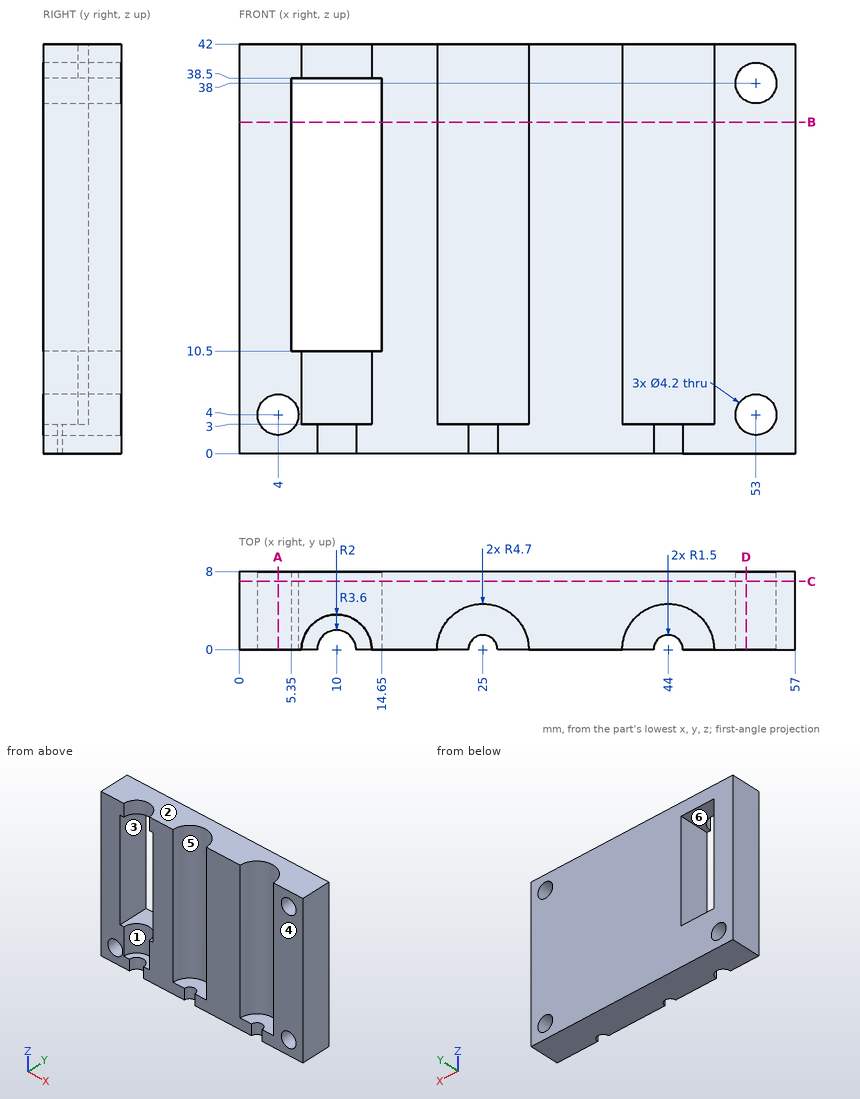
Print and shaded views of the part. All mm, measured from the part's lowest x, y and z. A direction names the side the tool comes from. Round coordinates to 2 decimals unless told otherwise and drop trailing zeros. Write each loop counter-clockwise with the first axis right and the second up, starting at its lowest first coordinate (ties: lowest second). Pieces come first, ordered by that corner, then holes.
(1) Probe line 1 along X through (y, z) = (5.5, 38); line 2 along X through (y, z) = (5, 4); line 3 along X through (y, z) = (2.25, 4). List the from-to ranges inside material, lowest first.
(2) Mould opens along Z. For the marked faces 1, 2 and 3 say: pulls with the +Z half, pulls with the -Z half, needs draft (parallel to the pull), parting line crosses it, or undercut.
(3) Slice it at D-D, the plane x = 52. Write the cut outline in (y, z).
(4) 3-axis set-ups, long thin cutter, end or side, ignore diameter. For the marked faces 4, 5 and 6: which of +Z, -Z, +X, -X, +Y, -Y reach the whole face in a straight line?
(5) Slice it at B-B, the plane z = 34. Write the cut outline in (x, y).
(6) Slice it at A-A, the plane x = 4. Write the cut outline in (y, z).
(7) Drop flat-ended pins along their axis: P1, Ø1.5, axis at x = 9.5, y = 6, coming from the -Z side; P2, Ø3.5, axis at x = 53, z = 4, coming from the +Y side; P3, Ø1.4, axis at x = 24, y = 2, coming from the +Z side. Give the stop position or say it passes through.
(8) Slice it at C-C, the plane y = 7. Write the cut outline in (x, z), and give its area (3 significant figures).
From the geometry:
1. line 1: x = 0 to 5.35, 14.65 to 50.9, 55.1 to 57
1. line 2: x = 0 to 1.9, 6.1 to 50.9, 55.1 to 57
1. line 3: x = 0 to 1.9, 6.1 to 7.19, 12.81 to 20.87, 29.13 to 39.87, 48.13 to 50.9, 55.1 to 57
2. face 1: needs draft
2. face 2: pulls with the +Z half
2. face 3: undercut
3. outline: (0, 0) - (8, 0) - (8, 2.15) - (0, 2.15) - close; (0, 5.85) - (8, 5.85) - (8, 36.15) - (0, 36.15) - close; (0, 39.85) - (8, 39.85) - (8, 42) - (0, 42) - close
4. face 4: +Z, -Z, +X, -X, -Y
4. face 5: +Z, -Y
4. face 6: +Y, -Y
5. outline: (0, 0) - (5.35, 0) - (5.35, 8) - (0, 8) - close; (14.65, 0) - (20.3, 0) arc R4.7 cw to (29.7, 0) - (39.3, 0) arc R4.7 cw to (48.7, 0) - (57, 0) - (57, 8) - (14.65, 8) - close
6. outline: (0, 0) - (8, 0) - (8, 1.9) - (0, 1.9) - close; (0, 6.1) - (8, 6.1) - (8, 42) - (0, 42) - close
7. P1: stops at z = 0
7. P2: passes through
7. P3: stops at z = 3
8. outline: (0, 0) - (57, 0) - (57, 42) - (0, 42) - close; hole circle Ø4.2 at (4, 4); hole (5.35, 10.5) - (14.65, 10.5) - (14.65, 38.5) - (5.35, 38.5) - close; hole circle Ø4.2 at (53, 4); hole circle Ø4.2 at (53, 38)
8. area: 2,090 mm2
